from build123d import *

# Parameters (mm, degrees)
SKETCH1_R           = 7
BOSS_EXTRUDE1_DEPTH = 65
SKETCH1_3_R         = 15
SKETCH1_3_R_2       = 7
BOSS_EXTRUDE2_DEPTH = 33
SKETCH3_W           = 30
SKETCH3_H           = 100
BOSS_EXTRUDE4_DEPTH = 10
SKETCH4_R           = 5
BOSS_EXTRUDE5_DEPTH = 15


with BuildPart() as part:
    # Sketch1 → Boss-Extrude1 (new body)
    with BuildSketch(Plane.XY):
        Circle(SKETCH1_R)
    extrude(amount=BOSS_EXTRUDE1_DEPTH)

    # Sketch1_3 → Boss-Extrude2 (add)
    with BuildSketch(Plane.XY):
        Circle(SKETCH1_3_R)
        Circle(SKETCH1_3_R_2, mode=Mode.SUBTRACT)
    extrude(amount=BOSS_EXTRUDE2_DEPTH)

    # Sketch3 → Boss-Extrude4 (add)
    with BuildSketch(Plane(origin=(0, 0, 0), x_dir=(-1, 0, 0), z_dir=(0, 0, -1))):
        Rectangle(SKETCH3_W, SKETCH3_H)
    extrude(amount=BOSS_EXTRUDE4_DEPTH)

    # Sketch4 → Boss-Extrude5 (add)
    with BuildSketch(Plane(origin=(0, 0, -10), x_dir=(-1, 0, 0), z_dir=(0, 0, -1))):
        with Locations(Location((0, -44.833870937, 0), (0, 0, 180))):
            Circle(SKETCH4_R)
    extrude(amount=BOSS_EXTRUDE5_DEPTH)


solid = part.part
Input: part model. Units: mm. Frame: model coordinates. A direction names the side the tool comes from. Round coordinates to 2 decimals unless told otherwise and drop trailing zeros. Order: outer loops, then holes, each group sorted by start corner. A loop starts at its lowest first (then second) coordinate and runs counter-clockwise, first axis right, second up.
1. Cut plane A-A, the plane x = 0. Output: boundary loops of the cut face in (y, z).
The answers:
outline: (-50, -10) - (-49.83, -10) - (-49.83, -25) - (-39.83, -25) - (-39.83, -10) - (50, -10) - (50, 0) - (15, 0) - (15, 33) - (7, 33) - (7, 65) - (-7, 65) - (-7, 33) - (-15, 33) - (-15, 0) - (-50, 0) - close
2. Set-up query: faces 1 (the face through (-1.08, -39.95, -17.4)), 2 (the face through (0, 50, -5)), 3 (the face through (6.466, -2.681, 48.776)). Return all of +Z, -Z, +X, -X, +Y, -Y with unobstructed straight access to the full face (end or side cutting, diameter ignored); none if empty.
The answers:
face 1: -Z
face 2: +Z, -Z, +X, -X, +Y
face 3: +Z
3. Cut plane C-C, the plane z = 45. Output: boundary loops of the cut face in (x, y), then the cut area to 3 significant figures.
The answers:
outline: circle Ø14 at (0, 0)
area: 154 mm2
4. Cut plane D-D, the plane z = 23. Output: boundary loops of the cut face in (x, y).
The answers:
outline: circle Ø30 at (0, 0)
5. Pin query (flat end, axial travel): P1, Ø8, axis at x = -9.5, z = 28, coming from the -Y side; P2, Ø9, axis at x = -2, y = -17, coming from the +Z side; P3, Ø6, axis at x = 8.5, z = 38, coming from the +Y side. Return the tip coordinate at first contact, or that it passes through.
The answers:
P1: stops at y = -13.96
P2: stops at z = 33
P3: stops at y = 4.33
6. Material intervals for line 1 (Z direction, x = -11.25, y = 28); line 2 (Z direction, x = 9.5, y = 6); line 3 (Y direction, x = 6, z = 43), sorted ascending.
The answers:
line 1: z = -10 to 0
line 2: z = -10 to 33
line 3: y = -3.61 to 3.61
7. Cut plane B-B, the plane y = 28.5. Output: boundary loops of the cut face in (x, z).
The answers:
outline: (-15, -10) - (15, -10) - (15, 0) - (-15, 0) - close
